Verification items for the finished model (mm, model axes). A direction names the side the tool comes from. Give positions to 0.01 mm unless a question says otherwise; leave off trailing zeros. Write each loop counter-clockwise with the first axis right and the second up, starting at its lowest first coordinate (ties: lowest second). Pieces come first, ordered by that corner, then holes. Notation, with made-up numbers: M 75.25,89.5 L 109.25,89.5 A16 cw 109.25,99.5 Z; hole C 28.5,-34.5 d10. An arc over 180 degrees is marked long. Write item = value, one per line.
from build123d import *

# Parameters (mm, degrees)
F0_R          = 12.7
F1_DEPTH      = 50.8
F2_R          = 10.3336081204
F3_DEPTH      = 37.592
F6_DEPTH      = 0.254
F7_R          = 2.54
F9_ANGLE_BACK = 2
F9_ANGLE      = 4


# Not quite as in the source:
# - a fillet or chamfer that OpenCascade refuses, or shapes differently, is made with other operations: its cross-section is extruded or revolved along the edge and cut away or added


with BuildPart() as f1:
    # F0 (on Front) → F1 (new body)
    with BuildSketch(Plane.XZ):
        Circle(F0_R)
    extrude(amount=F1_DEPTH)

    # F2 (on face) → F3 (cut)
    with BuildSketch(Plane.XZ.offset(50.8)):
        Circle(F2_R)
    extrude(amount=-F3_DEPTH, mode=Mode.SUBTRACT)

    # F8: F6 across plane


with BuildPart() as f6:
    # F5 (on Top) → F6 (new body, symmetric)
    with BuildSketch(Plane.XY):
        Polygon((-12.446, -31.75), (-12.446, 0), (-31.496, 0), align=None)
    extrude(amount=F6_DEPTH, both=True)

    # F7
    f7_edges = [f6.edges().sort_by_distance(p)[0] for p in [
        (-31.496, 0, 0),
    ]]
    fillet(f7_edges, radius=F7_R)


with BuildPart() as f1_1:
    add(f1.part)
    add(f6.part.mirror(Plane.YZ))

    # F4 (on Right) → F9 (revolve)
    with BuildSketch(Plane.YZ, mode=Mode.PRIVATE) as f9_sk:
        with BuildLine():
            Line((0, -12.192), (-35.6481084037, -12.192))
            add(Edge.make_bspline(
                [(-35.6481084037, -12.192), (-33.4311420603, -15.1893612741), (-28.0519206857, -33.0906197841), (-9.917521665, -17.0447887187), (0, -12.192)],
                knots=[0, 0, 0, 0, 0.4167760817, 1, 1, 1, 1], degree=3))
        make_face()
    revolve(f9_sk.sketch.rotate(Axis((0, 0, 0), (0, 1, 0)), -F9_ANGLE_BACK), axis=Axis((0, 0, 0), (0, 1, 0)), revolution_arc=F9_ANGLE)

    # F10: chamfer of 5.08 on 1 edges, made by hand

    # F10_s1 → F10_t2 (revolve, cut)
    with BuildSketch(Plane.XY):
        Polygon((12.7, -45.72), (7.62, -50.8), (12.7, -50.8), align=None)
    revolve(axis=Axis((0, -50.8, 0), (0, -1, 0)), mode=Mode.SUBTRACT)



with BuildPart() as f1_2:
    add(f1_1.part)

    add(f6.part)  # F11 merges F6
    # F11: F1 across plane
    add(f1_1.part.mirror(Plane.XY))


solid = f1_2.part
1) Tool access check on faces 5 (the flat face through (19, -12, -0.254)), 6 (the flat face through (0, 0, 0)), 7 (the flat face through (-19, -12, 0.254)), 8 (the cylindrical face through (-29.238, -1.321, -0.004)), 9 (the flat face through (19, -12, 0.254)). Record the directions out of +Z, -Z, +X, -X, +Y, -Y that give a thin tool (end or side, any length) a straight path to the whole face; none if there is none.
From the geometry:
face_5 = -Z, +X, +Y, -Y
face_6 = +Z, -Z, +X, -X, +Y
face_7 = +Z, -X, +Y, -Y
face_8 = +Z, -Z, -X
face_9 = +Z, +X, +Y, -Y
2) Cross-section at B-B on x = 20.5. Record the boundary of the cut face in (y, z), plus the area to 3 significant figures.
From the geometry:
outline = M -18.33,-0.25 L 0,-0.25 L 0,0.25 L -18.33,0.25 Z
area = 9.31 mm^2
3) Cross-section at A-A on x = -26. Record the boundary of the cut face in (y, z), plus the area to 3 significant figures.
From the geometry:
outline = M -9.16,-0.25 L 0,-0.25 L 0,0.25 L -9.16,0.25 Z
area = 4.65 mm^2
4) Draft check along Z on faces 1 (the cylindrical face through (-10.324, -30.891, 0.454)), 2 (the flat face through (-21.058, -17.396, 0.004)), 3 (the flat face through (-19, -12, -0.254)), 4 (the flat face through (0, -13.208, 0)). Enter one of: +Z half, -Z half, draft (parallel to the pull), parting line (faces both ways), or undercut.
From the geometry:
face_1 = undercut
face_2 = draft
face_3 = -Z half
face_4 = undercut
5) Material ranges on probe 1 along Z at (x, y) = (-24.5, -6); probe 2 along Y at (x, z) = (6, -6); probe 3 along X at (y, z) = (-33, -8), recorded low to high. Write a range as from..to.
From the geometry:
probe_1 = -0.25..0.25
probe_2 = -13.21..0
probe_3 = -9.86..-6.54, 6.54..9.86
6) Depth check by flat-ended pin: P1, Ø1.5, axis at y = -12.5, z = -7, coming from the +X side; P2, Ø18.5, axis at x = 0, z = 0, coming from the -Y side; P3, Ø3, axis at x = 0, y = -40, coming from the +Z side; P4, Ø1, axis at x = -15, y = -40.5, coming from the -Z side. Enter the tip coordinate at first touch or a pass-through.
From the geometry:
P1 = 11.06
P2 = -13.21
P3 = 12.7
P4 = through
